Geometry: final body of the model. Coordinates: model frame, mm. A direction names the side the tool comes from. Coordinates: 2 decimals unless noted, no trailing zeros. Order: outer loops, then holes, each group sorted by start corner. A loop starts at its lowest first (then second) coordinate and runs counter-clockwise, first axis right, second up. Notation, with made-up numbers: (38.5, -17) - (84.5, -17) arc R22 cw to (84.5, 20) - close; hole circle Ø1 at (13.25, 44.25). An arc over 180 degrees is marked (long way). Use one line per item in the form item = value. Start each with the question number.
Autodesk Inventor part; units mm, degrees
ref_plane "Work Plane1" through (0, 0, -15) normal (0, 0, 1) x (1, 0, 0)
ref_plane "YZ Plane" through (0, 0, 0) normal (1, 0, 0) x (0, 1, 0)
ref_plane "XZ Plane" through (0, 0, 0) normal (0, 1, 0) x (-1, 0, 0)
sketch "Sketch1" plane through (0, 0, 0) normal (0, 0, 1) x (1, 0, 0)
  line L0 (0, 0) -> (25, 0)
  line L1 (25, 0) -> (25, 40)
  line L2 (25, 40) -> (0, 40)
  line L3 (0, 40) -> (0, 0)
  dimension "d1" = 25
  dimension "d2" = 40
  dimension "d3" = 25
extrude "Extrusion1" add sketch "Sketch1" against normal blind 30
sketch "Sketch2" plane through (25, 0, 0) normal (1, 0, 0) x (0, 0, -1)
  line L0 (0, 0) -> (30, 0)
  circle A0 centre (15, 6.56) radius 2.46
extrude "Extrusion2" cut sketch "Sketch2" against normal blind 30
sketch "Sketch3" plane through (0, 0, 0) normal (-1, 0, 0) x (0, 0, 1)
  line L0 (0, 0) -> (-30, 0)
  line L1 (-25.05, 0) -> (-4.95, 0)
  line L2 (-4.95, 0) -> (-4.95, 33.12)
  line L3 (-4.95, 33.12) -> (-25.05, 33.12)
  line L4 (-25.05, 33.12) -> (-25.05, 0)
  dimension "d11" = 20.1
extrude "Extrusion3" cut sketch "Sketch3" against normal blind 20
sketch "Sketch4" plane through (0, 0, 0) normal (0, -1, 0) x (1, 0, 0)
  line L0 (20, -4.95) -> (20, -25.05)
  line L1 (20, -15) -> (25, -15)
  line L2 (25, 0) -> (25, -30)
  line L3 (20, -8.025) -> (25, -8.025)
  line L4 (25, -8.025) -> (25, -21.975)
  line L5 (25, -21.975) -> (20, -21.975)
  line L6 (20, -21.975) -> (20, -8.025)
  line L7 (20, -8.025) -> (25, -21.975) construction
  line L8 (25, -8.025) -> (20, -21.975) construction
  line L9 (25, -12.54) -> (25, -17.46)
  point P0 (0, 0)
  point P1 (22.5, -15)
  dimension "d14" = 13.95
extrude "Extrusion4" add sketch "Sketch4" along normal blind 15
sketch "Sketch5" plane through (20, 0, 0) normal (-1, 0, 0) x (0, 0, 1)
  circle A0 centre (-15, 6.56) radius 2.46
  circle A1 centre (-15, 6.56) radius 4.7025
  circle A2 centre (-15, 6.56) radius 2.46
  circle A3 centre (-15, 6.56) radius 2.46
  point P0 (0, 0)
  dimension "d17" = 9.405
extrude "Extrusion5" cut sketch "Sketch5" against normal blind 2.1
sketch "Sketch6" plane through (25, 0, 0) normal (1, 0, 0) x (0, 0, -1)
  circle A0 centre (15, 6.56) radius 4.7025
  line L0 (15, 6.56) -> (15, 23.56)
  circle A1 centre (15, 23.56) radius 2.46
  point P0 (0, 0)
  dimension "d20" = 17
  dimension "d21" = 4.92
extrude "Extrusion6" cut sketch "Sketch6" against normal blind 10 contours A1
sketch "Sketch7" plane through (20, 0, 0) normal (-1, 0, 0) x (0, 0, 1)
  circle A0 centre (-15, 23.56) radius 2.46
  circle A1 centre (-15, 23.56) radius 4.7025
  point P0 (0, 0)
  dimension "d24" = 9.405
extrude "Extrusion7" cut sketch "Sketch7" against normal blind 2.1
sketch "Sketch9" plane through (25, 0, 0) normal (1, 0, 0) x (0, 0, -1)
  circle A0 centre (15, 6.56) radius 2.46
  circle A1 centre (15, 6.56) radius 2.46
  circle A2 centre (15, 23.56) radius 2.46
  circle A3 centre (15, 23.56) radius 2.46
  line L0 (30, 40) -> (30, 0)
  line L1 (30, 0) -> (30, 40)
  line L2 (30, 40) -> (0, 40)
  line L3 (0, 40) -> (0, 0)
  line L4 (0, 0) -> (8.025, 0)
  line L5 (21.975, 0) -> (21.975, -15)
  line L6 (21.975, -15) -> (8.025, -15)
  line L7 (8.025, -15) -> (8.025, 0)
  line L8 (0, 0) -> (8.025, 0)
  line L9 (21.975, 0) -> (30, 0)
extrude "Extrusion8" add sketch "Sketch9" along normal blind 5
sketch "Sketch10" plane through (0, 40, 0) normal (0, 1, 0) x (1, 0, 0)
  line L0 (0, 30) -> (30, 30)
  line L1 (30, 0) -> (0, 0)
  line L2 (0, 30) -> (30, 30)
  line L3 (30, 30) -> (30, 0)
  line L4 (30, 0) -> (0, 0)
  line L5 (0, 0) -> (0, 30)
extrude "Extrusion9" add sketch "Sketch10" along normal blind 30
sketch "Sketch12" plane through (30, 0, 0) normal (1, 0, 0) x (0, 0, -1)
  circle A0 centre (15, 6.56) radius 2.46
  line L0 (15, 6.56) -> (15, 15.06)
  circle A1 centre (15, 15.06) radius 2.525
  point P0 (0, 0)
  dimension "d31" = 8.5
  dimension "d33" = 5.05
extrude "Extrusion10" cut sketch "Sketch12" against normal blind 30 contours A1
sketch "Sketch14" plane through (0, 0, 0) normal (0, 0, 1) x (1, 0, 0)
  line L0 (30, 70) -> (0, 70)
  line L1 (0, 100) -> (-8, 100)
  line L2 (30, 0) -> (30, 70)
  line L3 (30, 118) -> (30, 70)
  line L4 (30, 105) -> (30, 100)
  line L5 (0, 70) -> (30, 70)
  line L6 (0, 70) -> (0, 100)
  line L7 (15, 136) -> (30, 118)
  line L8 (-8, 136) -> (15, 136)
  line L9 (-8, 100) -> (-8, 136)
  point P0 (0, 0)
  dimension "d47" = 30
extrude "Extrusion12" add sketch "Sketch14" against normal blind 30
sketch "Sketch15" plane through (0, 0, -25.05) normal (-1, 0, 0) x (0, 0, 1)
  line L0 (0, 33.12) -> (20.1, 33.12)
  line L1 (20.1, 33.12) -> (20.1, 0)
  line L2 (0, 33.12) -> (20.1, 33.12)
  line L3 (20.1, 33.12) -> (20.1, 31.1)
  line L4 (20.1, 31.1) -> (0, 31.1)
  line L5 (0, 31.1) -> (0, 33.12)
  point P0 (25.05, 0)
  dimension "d57" = 2.02
extrude "Extrusion13" add sketch "Sketch15" against normal blind 20
sketch "Sketch23" plane through (0, 0, 0) normal (0, 0, 1) x (1, 0, 0)
  line L0 (0, 100) -> (-8, 100)
  line L1 (-8, 136) -> (15, 136)
  line L2 (-8, 136) -> (15, 136)
  line L3 (30, 118) -> (15, 136)
  line L4 (15, 136) -> (30, 118)
  line L5 (30, 118) -> (30, 93)
  line L6 (30, 0) -> (30, 118)
  line L7 (30, 93) -> (0, 93)
  line L8 (0, 93) -> (0, 100)
  line L9 (-8, 100) -> (0, 100)
  line L10 (15, 136) -> (-8, 136)
  line L11 (-8, 136) -> (-8, 100)
  point P0 (0, 0)
  point P1 (-2, 102)
  point P2 (4, 118)
  point P3 (-2, 134)
  dimension "d85" = 25
extrude "Extrusion14" add sketch "Sketch23" along normal blind 15
ref_plane "Work Plane1" through (0, 0, -15) normal (0, 0, 1) x (1, 0, 0)
mirror "Mirror1" about plane through (0, 0, -15) normal (0, 0, 1) of "Extrusion14"
sketch "Sketch30" plane through (-8, 136, 15) normal (0, 1, 0) x (1, 0, 0)
  line L0 (0, 60) -> (0, 0)
  line L1 (0, 30) -> (5, 30)
  line L2 (5, 30) -> (0, 0)
  line L3 (5, 30) -> (0, 60)
  line L4 (0, 60) -> (0, 0)
  point P0 (8, 15)
  dimension "d105" = 5
extrude "Extrusion18" cut sketch "Sketch30" against normal through all
properties part number "orien_b_50mm"
(1) Cut plane D-D on y = 103.5. Return the cut outline in (x, z), plus the area to 3 significant figures.
(2) Cut plane A-A on y = 15.06. Return the cut outline in (x, z) (3 decimals).
(3) Cut plane C-C on z = 3.5. Return the cut outline in (x, y).
(4) Material intervals for L1, parallel to Z at x = 25.25, y = 15.06 (3 decimals); L2, parallel to Y at x = 26, z = -15 (3 decimals); L3, parallel to Y at x = 14.5, z = 2.5, sorted ascending. Write a range as from..to.
(5) Contact query for flat-ended pins moving along their axis: pin 1 Ø12 at (x, z) = (14.5, -39.5) entering from -Y; pin 2 Ø16 at (y, z) = (17.5, -16) entering from -X; pin 3 Ø8 at (y, z) = (61, -11.5) entering from -X; pin 4 Ø1.5 at (y, z) = (45.5, 2) entering from +X. Output: stop coordinate, or through.
(6) Draft query along Z for faces 1 (the flat face through (25, -15, -15)), 2 (the cylindrical face through (25.995, 7.502, -17.272)), 3 (the flat face through (25, -8, -8.025)), 4 (the cylindrical face through (25.995, 24.502, -17.272)). Return one class per face: released by +Z, released by -Z, zero draft, split by the parting line, or undercut.
(7) Cut plane B-B on x = 18.5. Return the cut outline in (y, z).
(8) Set-up query: faces 5 (the flat face through (10, 16, -25.05)), 6 (the flat face through (15, 47, -30)), 7 (the flat face through (0, 62, -15)). Return all of +Z, -Z, +X, -X, +Y, -Y with unobstructed straight access to the full face (end or side cutting, diameter ignored); none if empty.
Check sheet entries:
q1.outline = (-8, -45) - (30, -45) - (30, 15) - (-8, 15) - (-3, -15) - close
q1.area = 2,130 mm^2
q2.outline = (0, -30) - (30, -30) - (30, -17.525) - (20, -17.525) - (20, -25.05) - (0, -25.05) - close; (0, -4.95) - (20, -4.95) - (20, -12.475) - (30, -12.475) - (30, 0) - (0, 0) - close
q3.outline = (-6.08, 100) - (0, 100) - (0, 93) - (30, 93) - (30, 118) - (15, 136) - (-6.08, 136) - close
q4.L1 = -30..-17.525, -12.475..0
q4.L2 = -15..4.1, 9.02..12.535, 17.585..21.1, 26.02..122.8
q4.L3 = 93..136
q5.pin_1 = 93
q5.pin_2 = 20
q5.pin_3 = 0
q5.pin_4 = through
q6.face_1 = zero draft
q6.face_2 = undercut
q6.face_3 = released by +Z
q6.face_4 = undercut
q7.outline = (0, -30) - (93, -30) - (93, -45) - (131.8, -45) - (131.8, 15) - (93, 15) - (93, 0) - (0, 0) - (0, -4.95) - (31.1, -4.95) - (31.1, -25.05) - (0, -25.05) - close
q8.face_5 = -X, -Y
q8.face_6 = -Z, +X, -X, -Y
q8.face_7 = +Z, -Z, -X, -Y
